Source: CAD feature listing. Evaluate the final solid. Frame: model axes, mm. A direction names the side the tool comes from. Give positions to 0.01 mm unless a question says otherwise; leave off trailing zeros. Loops run counter-clockwise (first coordinate to the right, second up) from the corner with the lowest first, then second, coordinate; pieces in that order, holes last.
```python
from build123d import *

# Parameters (mm, degrees)
SKETCH1_R           = 14.2875
SKETCH1_R_2         = 2.5527
BOSS_EXTRUDE1_DEPTH = 6.35


with BuildPart() as part:
    # Sketch1 → Boss-Extrude1 (new body)
    with BuildSketch(Plane.XY):
        with BuildLine():
            Line((14.189265695, 0), (138.210734305, 0))
            ThreePointArc((138.210734305, 0), (147.673860132, 4.230097428), (150.833057735, 14.102480381))
            Line((150.833057735, 14.102480381), (128.255279958, 217.302480381))
            ThreePointArc((128.255279958, 217.302480381), (124.102859099, 225.363125827), (115.632956527, 228.6))
            Line((115.632956527, 228.6), (36.767043473, 228.6))
            ThreePointArc((36.767043473, 228.6), (28.297140901, 225.363125827), (24.144720042, 217.302480381))
            Line((24.144720042, 217.302480381), (1.566942265, 14.102480381))
            ThreePointArc((1.566942265, 14.102480381), (4.726139868, 4.230097428), (14.189265695, 0))
        make_face()
        with Locations((76.2, 185.4708)):
            Circle(SKETCH1_R, mode=Mode.SUBTRACT)
        with Locations((94.160512242, 203.431312242)):
            Circle(SKETCH1_R_2, mode=Mode.SUBTRACT)
        with Locations((94.160512242, 167.510287758)):
            Circle(SKETCH1_R_2, mode=Mode.SUBTRACT)
        with Locations((58.239487758, 167.510287758)):
            Circle(SKETCH1_R_2, mode=Mode.SUBTRACT)
        with Locations((58.239487758, 203.431312242)):
            Circle(SKETCH1_R_2, mode=Mode.SUBTRACT)
        with BuildLine():
            Line((98.2218, 19.05), (98.2218, 31.75))
            ThreePointArc((98.2218, 31.75), (101.6, 35.1282), (104.9782, 31.75))
            Line((104.9782, 31.75), (104.9782, 19.05))
            ThreePointArc((104.9782, 19.05), (101.6, 15.6718), (98.2218, 19.05))
        make_face(mode=Mode.SUBTRACT)
        with BuildLine():
            Line((71.1581, 19.05), (71.1581, 31.75))
            ThreePointArc((71.1581, 31.75), (76.2, 36.7919), (81.2419, 31.75))
            Line((81.2419, 31.75), (81.2419, 19.05))
            ThreePointArc((81.2419, 19.05), (76.2, 14.0081), (71.1581, 19.05))
        make_face(mode=Mode.SUBTRACT)
        with BuildLine():
            Line((130.3782, 19.05), (130.3782, 31.75))
            ThreePointArc((130.3782, 31.75), (127, 35.1282), (123.6218, 31.75))
            Line((123.6218, 31.75), (123.6218, 19.05))
            ThreePointArc((123.6218, 19.05), (127, 15.6718), (130.3782, 19.05))
        make_face(mode=Mode.SUBTRACT)
        with BuildLine():
            Line((54.1782, 19.05), (54.1782, 31.75))
            ThreePointArc((54.1782, 31.75), (50.8, 35.1282), (47.4218, 31.75))
            Line((47.4218, 31.75), (47.4218, 19.05))
            ThreePointArc((47.4218, 19.05), (50.8, 15.6718), (54.1782, 19.05))
        make_face(mode=Mode.SUBTRACT)
        with BuildLine():
            Line((28.7782, 19.05), (28.7782, 31.75))
            ThreePointArc((28.7782, 31.75), (25.4, 35.1282), (22.0218, 31.75))
            Line((22.0218, 31.75), (22.0218, 19.05))
            ThreePointArc((22.0218, 19.05), (25.4, 15.6718), (28.7782, 19.05))
        make_face(mode=Mode.SUBTRACT)
        with BuildLine():
            Line((28.7782, 50.9524), (28.7782, 63.6524))
            ThreePointArc((28.7782, 63.6524), (25.4, 67.0306), (22.0218, 63.6524))
            Line((22.0218, 63.6524), (22.0218, 50.9524))
            ThreePointArc((22.0218, 50.9524), (25.4, 47.5742), (28.7782, 50.9524))
        make_face(mode=Mode.SUBTRACT)
        with BuildLine():
            Line((54.1782, 50.9524), (54.1782, 63.6524))
            ThreePointArc((54.1782, 63.6524), (50.8, 67.0306), (47.4218, 63.6524))
            Line((47.4218, 63.6524), (47.4218, 50.9524))
            ThreePointArc((47.4218, 50.9524), (50.8, 47.5742), (54.1782, 50.9524))
        make_face(mode=Mode.SUBTRACT)
        with BuildLine():
            Line((81.2419, 50.9524), (81.2419, 63.6524))
            ThreePointArc((81.2419, 63.6524), (76.2, 68.6943), (71.1581, 63.6524))
            Line((71.1581, 63.6524), (71.1581, 50.9524))
            ThreePointArc((71.1581, 50.9524), (76.2, 45.9105), (81.2419, 50.9524))
        make_face(mode=Mode.SUBTRACT)
        with BuildLine():
            Line((104.9782, 50.9524), (104.9782, 63.6524))
            ThreePointArc((104.9782, 63.6524), (101.6, 67.0306), (98.2218, 63.6524))
            Line((98.2218, 63.6524), (98.2218, 50.9524))
            ThreePointArc((98.2218, 50.9524), (101.6, 47.5742), (104.9782, 50.9524))
        make_face(mode=Mode.SUBTRACT)
        with BuildLine():
            Line((123.6218, 50.9524), (123.6218, 63.6524))
            ThreePointArc((123.6218, 63.6524), (127, 67.0306), (130.3782, 63.6524))
            Line((130.3782, 63.6524), (130.3782, 50.9524))
            ThreePointArc((130.3782, 50.9524), (127, 47.5742), (123.6218, 50.9524))
        make_face(mode=Mode.SUBTRACT)
    extrude(amount=BOSS_EXTRUDE1_DEPTH)


solid = part.part
```
(1) Ray query, line 1 along Y through (x, z) = (76.2, 3.5); line 2 along Y through (x, z) = (116, 4.75); line 3 along Y through (x, z) = (53, 6.25). Return the intervals inside material, ascending.
A:
line 1: y = 0 to 14.01, 36.79 to 45.91, 68.69 to 171.18, 199.76 to 228.6
line 2: y = 0 to 228.59
line 3: y = 0 to 16.49, 34.31 to 48.39, 66.22 to 228.6
(2) Section A-A, the plane y = 196. Return the cut outline in (x, z).
A:
outline: (21.78, 0) - (66.54, 0) - (66.54, 6.35) - (21.78, 6.35) - close; (85.86, 0) - (130.62, 0) - (130.62, 6.35) - (85.86, 6.35) - close
(3) Section D-D, the plane z = 4. Count the separate pieces of the cut face and the enclosed holes in it, then the cut area to 3 significant figures.
A:
separate pieces: 1
enclosed holes: 15
area: 26,800 mm2
(4) Section C-C, the plane x = 50.8. Return the cut outline in (y, z), then the cut area to 3 significant figures.
A:
outline: (0, 0) - (15.67, 0) - (15.67, 6.35) - (0, 6.35) - close; (35.13, 0) - (47.57, 0) - (47.57, 6.35) - (35.13, 6.35) - close; (67.03, 0) - (228.6, 0) - (228.6, 6.35) - (67.03, 6.35) - close
area: 1,200 mm2
(5) Mould query, pull axis X, two halves, no side actions, for faces 3 (the cylindrical face through (4.63, 4.34, 3.13)), 4 (the cylindrical face through (101.674, 15.673, 3.131)), 5 (the cylindrical face through (147.574, 4.119, 3.131)). Classes: pulls with the +X half, pulls with the -X half, needs draft (parallel to the pull), parting line crosses it, or undercut.
A:
face 3: pulls with the -X half
face 4: undercut
face 5: pulls with the +X half
(6) Section B-B, the plane x = 76.2. Return the cut outline in (y, z).
A:
outline: (0, 0) - (14.01, 0) - (14.01, 6.35) - (0, 6.35) - close; (36.79, 0) - (45.91, 0) - (45.91, 6.35) - (36.79, 6.35) - close; (68.69, 0) - (171.18, 0) - (171.18, 6.35) - (68.69, 6.35) - close; (199.76, 0) - (228.6, 0) - (228.6, 6.35) - (199.76, 6.35) - close
(7) Reachability of faces 1 (the flat face through (75, 0, 3)), 2 (the cylindrical face through (101.526, 35.127, 3.131)) from +Z, -Z, +X, -X, +Y, -Y: full face, straight path, thin tool, end or side. Return the list, or none.
A:
face 1: +Z, -Z, +X, -X, -Y
face 2: +Z, -Z
(8) First-contact query: pin 1 (3 mm diameter, centred on y = 54.5, z = 4, fed in from +X); pin 2 (4 mm diameter, centred on x = 58.24, y = 167.51, fed in from -Z); pin 3 (3 mm diameter, centred on y = 57.5, z = 3, fed in from -X); pin 4 (1.9 mm diameter, centred on y = 60, z = 4, fed in from +X). Flat tips, straight axial feed; report the tip coordinate or a pass-through.
A:
pin 1: stops at x = 146.51
pin 2: passes through
pin 3: stops at x = 6.22
pin 4: stops at x = 145.84
